from build123d import *

# Parameters (mm, degrees)
F1_DEPTH = 50.8
F2_W     = 342.9
F2_H     = 76.2
F3_DEPTH = 127


with BuildPart() as f1:
    # F0 (on Top) → F1 (new body)
    with BuildSketch(Plane.XY):
        with BuildLine():
            Line((155.575, 117.475), (-155.575, 117.475))
            ThreePointArc((-155.575, 117.475), (-157.820064, 116.545064), (-158.75, 114.3))
            Line((-158.75, 114.3), (-158.75, 33.901519))
            ThreePointArc((-158.75, 33.901519), (-55.013583, -14.281315), (-2.091765, -115.682059))
            ThreePointArc((-2.091765, -115.682059), (0, -117.475), (2.091765, -115.682059))
            ThreePointArc((2.091765, -115.682059), (55.013583, -14.281315), (158.75, 33.901519))
            Line((158.75, 33.901519), (158.75, 114.3))
            ThreePointArc((158.75, 114.3), (157.820064, 116.545064), (155.575, 117.475))
        make_face()
    extrude(amount=-F1_DEPTH)

    # F2 (on Front) → F3 (cut, symmetric)
    with BuildSketch(Plane.XZ):
        with Locations((0, -25.4)):
            Rectangle(F2_W, F2_H)
        with BuildLine():
            Line((158.75, -50.8), (-158.75, -50.8))
            Line((-158.75, -50.8), (-158.75, -30.059666))
            ThreePointArc((-158.75, -30.059666), (-157.527006, -26.31316), (-154.329114, -24.009789))
            ThreePointArc((-154.329114, -24.009789), (0, 0), (154.329114, -24.009789))
            ThreePointArc((154.329114, -24.009789), (157.527006, -26.31316), (158.75, -30.059666))
            Line((158.75, -30.059666), (158.75, -50.8))
        make_face(mode=Mode.SUBTRACT)
    extrude(amount=F3_DEPTH, both=True, mode=Mode.SUBTRACT)


solid = f1.part
Here's how the part is built. I have some questions about the finished solid (model axes, mm). Coordinates: 2 decimals unless noted, no trailing zeros. Write each loop counter-clockwise with the first axis right and the second up, starting at its lowest first coordinate (ties: lowest second). Pieces come first, ordered by that corner, then holes. Notation, with made-up numbers: (-32, 23.5) - (-26, 23.5) arc R22 ccw to (-26, 53.5) - close; hole circle Ø8 at (-23, 5.5). An arc over 180 degrees is marked (long way). Use one line per item in the form item = value.
1) I'm going to push flat-ended pins straight in: P1, Ø4, axis at y = -92, z = -23, coming from the +X side; P2, Ø8, axis at x = -122.5, z = -7, coming from the -Y side; P3, Ø8, axis at x = 39.5, z = -9.5, coming from the -Y side; P4, Ø1.5, axis at x = 14.5, y = -59, coming from the +Z side. Where does each tip first touch, or does it pass through?
Solved:
P1 = 8.04
P2 = through
P3 = -36.28
P4 = -0.19
2) I need wall thicknesses on line 1 (Y direction, x = -72, z = -20) (3 decimals); line 2 (Z direction, x = 114, y = 91); line 3 (Z direction, x = -25, y = 76). Which ranges of each line are inside material? Lowest first, please.
Solved:
line_1 = 0.021 to 117.475
line_2 = -50.8 to -12.96
line_3 = -50.8 to -0.62
3) Thinking about a two-plate mould opening in X: for faces 1 (the cylindrical face through (-56.2, -13.16, -25.05)), 2 (the cylindrical face through (-2.195, 50.566, -0.005)), 3 (the flat face through (-2, 54, -50.8)), which applies, released by +X, released by -X, zero draft, split by the parting line, or undercut?
Solved:
face_1 = released by -X
face_2 = split by the parting line
face_3 = zero draft
4) Suppose I cut it at A-A, the plane z = -17. Write out the boundary of the cut face in (x, y) (3 decimals).
Solved:
outline = (-130.319, 28.468) arc R177.8 cw to (-2.092, -115.682) arc R2.117 ccw to (2.092, -115.682) arc R177.8 cw to (130.319, 28.468) - (130.319, 117.475) - (-130.319, 117.475) - close
5) Suppose I cut it at B-B, the plane x = 63.5. Write out the boundary of the cut face in (y, z) (3 decimals), plus the area to 3 significant figures.
Solved:
outline = (-6.683, -50.8) - (117.475, -50.8) - (117.475, -3.984) - (-6.683, -3.984) - close
area = 5,810 mm2
6) Suppose I cut it at C-C, the plane y = 1.5. Write out the boundary of the cut face in (x, z), plus the area to 3 significant figures.
Solved:
outline = (-74.03, -50.8) - (74.03, -50.8) - (74.03, -5.42) arc R508 ccw to (-74.03, -5.42) - close
area = 7,250 mm2
